The model under review builds one solid part; all positions refer to its coordinate system, in mm. Face numbers are marked on the shaded views. A direction names the side the tool comes from. Give positions to 0.01 mm unless a question says otherwise; leave off trailing zeros. Order: outer loops, then holes, each group sorted by start corner. A loop starts at its lowest first (then second) coordinate and runs counter-clockwise, first axis right, second up. Notation, with made-up numbers: (13, 35.5) -> (32, 35.5) arc R22 cw to (32, 60.5) -> close; hole circle Ø7 at (52.5, 51.25). An arc over 180 degrees is marked (long way). Answer as a JSON object with one key per item and string values. Group by question number.
from build123d import *

# Parameters (mm, degrees)
F2_W     = 50
F2_H     = 60
F0_W     = 50
F0_H     = 50
F4_W     = 40
F4_H     = 60
F5_DEPTH = 50
F6_R     = 13.75
F7_DEPTH = 25.4


with BuildPart() as f3:
    # F2 (on offset) → F3 section 0
    with BuildSketch(Plane.XZ.offset(-70)):
        with Locations((0, -5)):
            Rectangle(F2_W, F2_H)
    # F0 (on Front) → F3 section 1
    with BuildSketch(Plane.XZ):
        Rectangle(F0_W, F0_H)
    loft()

    # F4 (on face) → F5 (cut)
    with BuildSketch(Plane.XY.offset(25)):
        with Locations((0, 35)):
            Rectangle(F4_W, F4_H)
    extrude(amount=-F5_DEPTH, mode=Mode.SUBTRACT)

    # F6 (on face) → F7 (cut)
    with BuildSketch(Plane.XZ):
        Circle(F6_R)
    extrude(amount=-F7_DEPTH, mode=Mode.SUBTRACT)


solid = f3.part
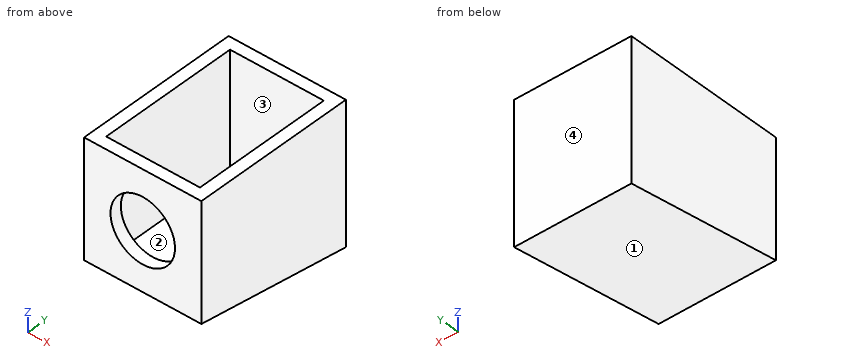
1. Machinability: for the marked faces 1 and 2, which of the approach directions +Z, -Z, +X, -X, +Y, -Y give a long, thin tool a straight path to every point of the face, cutting with its end or side? Answer none if there is none.
2. Take a section at B-B on x = -17. Give the boundary of the cut face in (y, z), plus the area to 3 significant figures.
3. Take a section at C-C on x = 5.5. Give the boundary of the cut face in (y, z), plus the area to 3 significant figures.
4. For pin 1 (25 mm diameter, centred on x = 0, z = 0, fed in from -Y); pin 2 (6 mm diameter, centred on x = 15.5, y = 22.5, fed in from -Z); pin 3 (20 mm diameter, centred on x = -5.5, y = 26, fed in from +Z), all flat-tipped, find the tip position at first contact; note any pin that passes through.
5. For probe 1 along Y at (x, z) = (9, -20.5); probe 2 along X at (y, z) = (39, -12); probe 3 along Z at (x, y) = (0, 2.55), list the stretches that pass through material, from the lowest coordinate up. Write a range as [from, to].
6. Draft analysis for pull direction X (two halves, no side actions). For the marked faces 3 and 4, state which applies: pulls with the +X half, pulls with the -X half, needs draft (parallel to the pull), parting line crosses it, or undercut.
7. Take a section at A-A on x = 0. Give the boundary of the cut face in (y, z).
Checks:
{
 "1": {"face 1": "-Z, +X, -X, -Y", "face 2": "+Z"},
 "2": {"outline": "(0, -25) -> (70, -35) -> (70, 25) -> (65, 25) -> (65, -25) -> (5, -25) -> (5, 25) -> (0, 25) -> close", "area": "850 mm2"},
 "3": {"outline": "(0, -25) -> (70, -35) -> (70, 25) -> (65, 25) -> (65, -25) -> (5, -25) -> (5, -12.6) -> (0, -12.6) -> close; (0, 12.6) -> (5, 12.6) -> (5, 25) -> (0, 25) -> close", "area": "724 mm2"},
 "4": {"pin 1": "stops at y = 65", "pin 2": "stops at z = -28.64", "pin 3": "stops at z = -25"},
 "5": {"probe 1": "y = [0, 5], [65, 70]", "probe 2": "x = [-25, -20], [20, 25]", "probe 3": "z = [-25.36, -13.75], [13.75, 25]"},
 "6": {"face 3": "undercut", "face 4": "needs draft"},
 "7": {"outline": "(0, -25) -> (70, -35) -> (70, 25) -> (65, 25) -> (65, -25) -> (5, -25) -> (5, -13.75) -> (0, -13.75) -> close; (0, 13.75) -> (5, 13.75) -> (5, 25) -> (0, 25) -> close"}
}
